```python
from build123d import *

# Parameters (mm, degrees)
SKETCH1_W           = 3.175
SKETCH1_H           = 29.34469697
BOSS_EXTRUDE1_DEPTH = 19.05
SKETCH2_W           = 3.175
SKETCH2_H           = 10.29469697
CUT_EXTRUDE1_DEPTH  = 5.08


with BuildPart() as part:
    # Sketch1 → Boss-Extrude1 (new body)
    with BuildSketch(Plane.XY):
        with Locations((82.43330737, 77.753797109)):
            Rectangle(SKETCH1_W, SKETCH1_H)
    extrude(amount=-BOSS_EXTRUDE1_DEPTH)

    # Sketch2 → Cut-Extrude1 (cut)
    with BuildSketch(Plane(origin=(84.02080737, 0, 0), x_dir=(0, 0, -1), z_dir=(1, 0, 0))):
        with Locations((1.5875, 77.753797109)):
            Rectangle(SKETCH2_W, SKETCH2_H)
        with Locations((17.4625, 77.753797109)):
            Rectangle(SKETCH2_W, SKETCH2_H)
    extrude(amount=-CUT_EXTRUDE1_DEPTH, mode=Mode.SUBTRACT)


solid = part.part
```
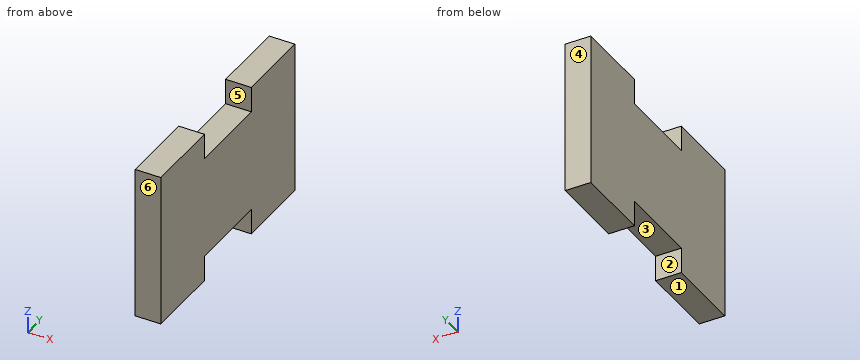
The listing builds one solid part. Answer for the finished solid, in the listing's coordinates (mm). Face numbers are marked on the shaded views. A direction names the side the tool comes from. Coordinates: 2 decimals unless noted, no trailing zeros. Write each loop counter-clockwise with the first axis right and the second up, starting at its lowest first coordinate (ties: lowest second). Pieces come first, ordered by that corner, then holes. Notation, with made-up numbers: M 25.25,-36.75 L 72.25,-36.75 A8 ccw 72.25,-32.75 Z; hole C 35.5,11 d8. An arc over 180 degrees is marked long. Use a Markdown table: item, result. Add a question column.
1. Section A-A (z = -17.5) is taken. Give the vertices of the cut face in (x, y), plus the area to 3 significant figures.
2. Section B-B (x = 83.35) is taken. Give the vertices of the cut face in (y, z) (3 decimals).
3. For a pull along Y with two mould halves and no side action, classify the marked faces 1, 2, 3 and 4 as +Y half, -Y half, draft (parallel to the pull), parting line (faces both ways), or undercut.
4. Which of the six approach directions +Z, -Z, +X, -X, +Y, -Y give full straight-line access (tool end or side, diameter ignored) to the marked faces 5 and 6?
5. Straight lines are drawn through the part: line 1 along Y through (x, z) = (81.65, -18); line 2 along Z through (x, y) = (82.55, 77) (3 decimals). For each, find the intervals that lie inside material, in ascending order. Write a range as [from, to].
6. Section C-C (y = 80.25) is taken. Give the vertices of the cut face in (x, z) (3 decimals).
Data:
| question | item | result |
|---|---|---|
| 1 | outline | M 80.85,63.08 L 84.02,63.08 L 84.02,72.61 L 80.85,72.61 Z; M 80.85,82.9 L 84.02,82.9 L 84.02,92.43 L 80.85,92.43 Z |
| 1 | area | 60.5 mm2 |
| 2 | outline | M 63.081,-19.05 L 72.606,-19.05 L 72.606,-15.875 L 82.901,-15.875 L 82.901,-19.05 L 92.426,-19.05 L 92.426,0 L 82.901,0 L 82.901,-3.175 L 72.606,-3.175 L 72.606,0 L 63.081,0 Z |
| 3 | face 1 | draft |
| 3 | face 2 | undercut |
| 3 | face 3 | undercut |
| 3 | face 4 | +Y half |
| 4 | face 5 | +Z, +X, -X |
| 4 | face 6 | +Z, -Z, +X, -X, -Y |
| 5 | line 1 | y = [63.08, 72.61], [82.9, 92.43] |
| 5 | line 2 | z = [-15.875, -3.175] |
| 6 | outline | M 80.846,-15.875 L 84.021,-15.875 L 84.021,-3.175 L 80.846,-3.175 Z |
